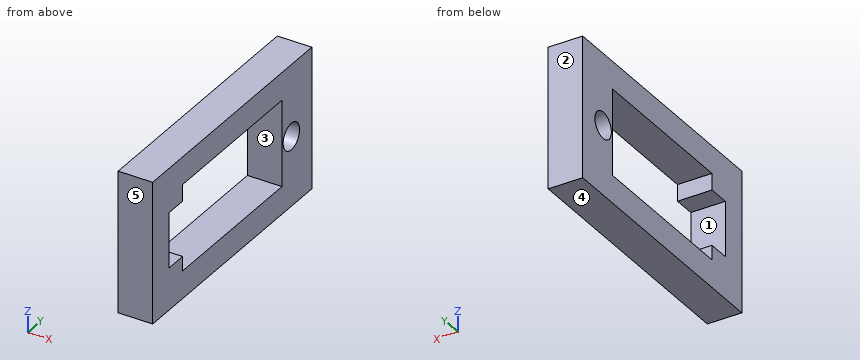
```python
from build123d import *

# Parameters (mm, degrees)
SKETCH1_W           = 20.5
SKETCH1_H           = 37.3
SKETCH1_W_2         = 12.5
SKETCH1_H_2         = 23.3
BOSS_EXTRUDE1_DEPTH = 5
SKETCH2_R           = 1.92
CUT_EXTRUDE1_DEPTH  = 13
SKETCH4_W           = 8
SKETCH4_H           = 3.126799126
CUT_EXTRUDE3_DEPTH  = 20


with BuildPart() as part:
    # Sketch1 → Boss-Extrude1 (new body)
    with BuildSketch(Plane(origin=(0, 0, 0), x_dir=(0, 0, -1), z_dir=(1, 0, 0))):
        with Locations((-0.15, -0.4)):
            Rectangle(SKETCH1_W, SKETCH1_H)
        with Locations((-0.15, -0.4)):
            Rectangle(SKETCH1_W_2, SKETCH1_H_2, mode=Mode.SUBTRACT)
    extrude(amount=BOSS_EXTRUDE1_DEPTH)

    # Sketch2 → Cut-Extrude1 (cut)
    with BuildSketch(Plane(origin=(5, 0, 0), x_dir=(0, 0, -1), z_dir=(1, 0, 0))):
        with Locations((0, 13.45)):
            Circle(SKETCH2_R)
    extrude(amount=-CUT_EXTRUDE1_DEPTH, mode=Mode.SUBTRACT)

    # Sketch4 → Cut-Extrude3 (cut)
    with BuildSketch(Plane(origin=(5, 0, 0), x_dir=(0, 0, -1), z_dir=(1, 0, 0))):
        with Locations((0, -13.613399563)):
            Rectangle(SKETCH4_W, SKETCH4_H)
    extrude(amount=-CUT_EXTRUDE3_DEPTH, mode=Mode.SUBTRACT)


solid = part.part
```
Design review of the part built by this model. Coordinates are the model's own, in mm. Face numbers are marked on the shaded views. A direction names the side the tool comes from. Round coordinates to 2 decimals unless told otherwise and drop trailing zeros. Write each loop counter-clockwise with the first axis right and the second up, starting at its lowest first coordinate (ties: lowest second). Pieces come first, ordered by that corner, then holes. Notation, with made-up numbers: (-2.5, 48.25) -> (17.5, 48.25) arc R29 cw to (17.5, 75.25) -> close; hole circle Ø6 at (44, -8). An arc over 180 degrees is marked (long way). Answer in a Markdown table with one row per item.
Q1. Take a section at A-A, the plane z = 0. State the section outline as (x, y) points, then the cut area to 3 significant figures.
The answers:
| item | result |
|---|---|
| outline | (0, -19.05) -> (5, -19.05) -> (5, -15.18) -> (0, -15.18) -> close; (0, 11.25) -> (5, 11.25) -> (5, 11.53) -> (0, 11.53) -> close; (0, 15.37) -> (5, 15.37) -> (5, 18.25) -> (0, 18.25) -> close |
| area | 35.2 mm² |
Q2. To check wall thickness, follow L1, parallel to Y at x = 3.3, z = 0; L2, parallel to Z at x = 3, y = 6; L3, parallel to Y at x = 0.95, z = 2.75. State the ranges of each line that lie inside material, in increasing order. Write a range as [from, to].
The answers:
| item | result |
|---|---|
| L1 | [-19.05, -15.18], [11.25, 11.53], [15.37, 18.25] |
| L2 | [-10.1, -6.1], [6.4, 10.4] |
| L3 | [-19.05, -15.18], [11.25, 18.25] |
Q3. For the marked faces 1 and 2, list the 3-axis set-ups (+Z, -Z, +X, -X, +Y, -Y) from which the entire face can be reached by the end or side of a thin tool; tool diameter is ignored.
The answers:
| item | result |
|---|---|
| face 1 | +X, -X |
| face 2 | +Z, -Z, +X, -X, +Y |
Q4. Take a section at C-C, the plane x = 3.65. State the section outline as (y, z) points, then the cut area to 3 significant figures.
The answers:
| item | result |
|---|---|
| outline | (-19.05, -10.1) -> (18.25, -10.1) -> (18.25, 10.4) -> (-19.05, 10.4) -> close; hole (-15.18, -4) -> (-12.05, -4) -> (-12.05, -6.1) -> (11.25, -6.1) -> (11.25, 6.4) -> (-12.05, 6.4) -> (-12.05, 4) -> (-15.18, 4) -> close; hole circle Ø3.84 at (13.45, 0) |
| area | 437 mm² |
Q5. Clearance check with a flat-ended pin moving along its axis: pin 1 Ø1 at (y, z) = (-12.5, -4.5) entering from -X. State where the tip first meets the part, or that it passes through.
The answers:
| item | result |
|---|---|
| pin 1 | x = 0 |
Q6. Take a section at D-D, the plane y = 13.45. State the section outline as (x, z) points, then the cut area to 3 significant figures.
The answers:
| item | result |
|---|---|
| outline | (0, -10.1) -> (5, -10.1) -> (5, -1.92) -> (0, -1.92) -> close; (0, 1.92) -> (5, 1.92) -> (5, 10.4) -> (0, 10.4) -> close |
| area | 83.3 mm² |
Q7. Draft analysis for pull direction Y (two halves, no side actions). For the marked faces 3, 4 and 5, state which applies: +Y half, -Y half, draft (parallel to the pull), parting line (faces both ways), or undercut.
The answers:
| item | result |
|---|---|
| face 3 | undercut |
| face 4 | draft |
| face 5 | -Y half |
Q8. Take a section at B-B, the plane y = -13. State the section outline as (x, z) points, then the cut area to 3 significant figures.
The answers:
| item | result |
|---|---|
| outline | (0, -10.1) -> (5, -10.1) -> (5, -4) -> (0, -4) -> close; (0, 4) -> (5, 4) -> (5, 10.4) -> (0, 10.4) -> close |
| area | 62.5 mm² |
